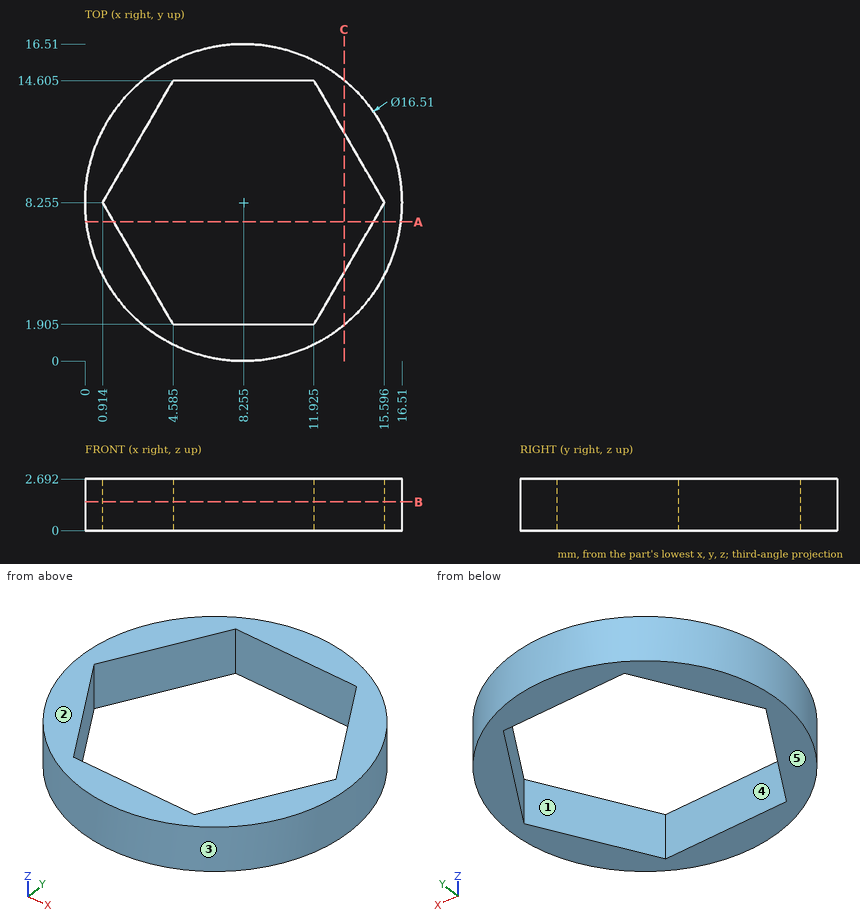
Answer from the drawing. Dimensions are ordinates in mm from the lowest x, y and z of the part. A direction names the side the tool comes from. Coordinates: 2 decimals unless noted, no trailing zeros. Order: outer loops, then holes, each group sorted by start corner. A loop starts at its lowest first (then second) coordinate and runs counter-clockwise, first axis right, second up. Notation, with made-up numbers: (1.25, 83) - (6.25, 83) arc R22 ccw to (6.25, 101) - close; hole circle Ø4 at (-40, -11). An arc over 180 degrees is marked (long way). Use one line per item in the form item = value.
(1) Given pin 1 Ø0.8 at (x, z) = (7, 1.5) entering from +Y; pin 2 Ø1.3 at (x, z) = (7, 0.5) entering from -Y; pin 3 Ø2 at (x, y) = (11.5, 9.5) entering from +Z; pin 4 Ø1.5 at (y, z) = (5, 1) entering from -X, each flat-ended and moving along its own axis, determine where each tip first touches the part or whether it passes through.
Computed values:
pin_1 = 16.47
pin_2 = 0.02
pin_3 = through
pin_4 = 0.39
(2) Section A-A, the plane y = 7.25 is taken. Give the vertices of the cut face in (x, z) (1 decimal).
Computed values:
outline = (0.1, 0) - (1.5, 0) - (1.5, 2.7) - (0.1, 2.7) - close; (15, 0) - (16.4, 0) - (16.4, 2.7) - (15, 2.7) - close
(3) Section C-C, the plane x = 13.5 is taken. Give the vertices of the cut face in (y, z), then the cut area to 3 significant figures.
Computed values:
outline = (1.88, 0) - (4.63, 0) - (4.63, 2.69) - (1.88, 2.69) - close; (11.88, 0) - (14.63, 0) - (14.63, 2.69) - (11.88, 2.69) - close
area = 14.8 mm²
(4) Which of the six approach directions +Z, -Z, +X, -X, +Y, -Y give full straight-line access (tool end or side, diameter ignored) to the marked faces 1 and 2?
Computed values:
face_1 = +Z, -Z
face_2 = +Z, +X, -X, +Y, -Y
(5) For a pull along X with two mould halves and no side action, classify the marked faces 3, 4 and 5 as pulls with the +X half, pulls with the -X half, needs draft (parallel to the pull), parting line crosses it, or undercut.
Computed values:
face_3 = parting line crosses it
face_4 = undercut
face_5 = needs draft
(6) Straight lines are drawn through the part: L1, parallel to Y at x = 8.5, z = 1.7 (1 decimal); L2, parallel to Y at x = 5, z = 2.65 (1 decimal); L3, parallel to X at y = 6.5, z = 1.7. For each, find the intervals that lie inside material, in ascending order.
Computed values:
L1 = 0 to 1.9, 14.6 to 16.5
L2 = 0.7 to 1.9, 14.6 to 15.8
L3 = 0.19 to 1.93, 14.58 to 16.32
(7) Section B-B, the plane z = 1.5 is taken. Give the vertices of the cut face in (x, y) (1 decimal).
Computed values:
outline = circle Ø16.5 at (8.3, 8.3); hole (0.9, 8.3) - (4.6, 1.9) - (11.9, 1.9) - (15.6, 8.3) - (11.9, 14.6) - (4.6, 14.6) - close
